```python
from build123d import *

# Parameters (mm, degrees)
SKETCH1_W           = 620
SKETCH1_H           = 680
BOSS_EXTRUDE1_DEPTH = 15
SKETCH2_R           = 4
CUT_EXTRUDE1_DEPTH  = 10
LPATTERN1_COUNT     = 3
LPATTERN1_PITCH     = 295
SKETCH3_R           = 4
CUT_EXTRUDE2_DEPTH  = 10
LPATTERN2_COUNT     = 3
LPATTERN2_PITCH     = 325
SKETCH7_R           = 4
CUT_EXTRUDE7_DEPTH  = 10
SKETCH8_W           = 10
SKETCH8_H           = 20
CUT_EXTRUDE8_DEPTH  = 435


with BuildPart() as part:
    # Sketch1 → Boss-Extrude1 (new body)
    with BuildSketch(Plane(origin=(0, 0, 0), x_dir=(0, 0, -1), z_dir=(1, 0, 0))):
        with Locations((0, 340)):
            Rectangle(SKETCH1_W, SKETCH1_H)
    extrude(amount=BOSS_EXTRUDE1_DEPTH)

    # Sketch2 → Cut-Extrude1 (cut)
    with BuildSketch(Plane.ZY):
        with Locations((295, 7.5)):
            Circle(SKETCH2_R)
    cut_extrude1 = extrude(amount=-CUT_EXTRUDE1_DEPTH, mode=Mode.SUBTRACT)

    # LPattern1: Cut-Extrude1 ×3
    with Locations(*[(0, 0, -i * LPATTERN1_PITCH) for i in range(1, LPATTERN1_COUNT)]):
        add(cut_extrude1, mode=Mode.SUBTRACT)

    # Sketch3 → Cut-Extrude2 (cut)
    with BuildSketch(Plane(origin=(0, 0, -310), x_dir=(-1, 0, 0), z_dir=(0, 0, -1))):
        with Locations((-7.5, 15)):
            Circle(SKETCH3_R)
    cut_extrude2 = extrude(amount=-CUT_EXTRUDE2_DEPTH, mode=Mode.SUBTRACT)

    # LPattern2: Cut-Extrude2 ×3
    with Locations(*[(0, i * LPATTERN2_PITCH, 0) for i in range(1, LPATTERN2_COUNT)]):
        add(cut_extrude2, mode=Mode.SUBTRACT)

    # Sketch7 → Cut-Extrude7 (cut)
    with BuildSketch(Plane.XY.offset(310)):
        with Locations((7.5, 670)):
            Circle(SKETCH7_R)
    extrude(amount=-CUT_EXTRUDE7_DEPTH, mode=Mode.SUBTRACT)

    # Sketch8 → Cut-Extrude8 (cut)
    with BuildSketch(Plane(origin=(0, 680, 0), x_dir=(1, 0, 0), z_dir=(0, 1, 0))):
        with Locations((10, -287.5)):
            Rectangle(SKETCH8_W, SKETCH8_H)
    extrude(amount=-CUT_EXTRUDE8_DEPTH, mode=Mode.SUBTRACT)


solid = part.part
```
Can you work these out from the model? Positions are in its coordinate system, mm. Give positions to 0.01 mm unless a question says otherwise; leave off trailing zeros. Write each loop counter-clockwise with the first axis right and the second up, starting at its lowest first coordinate (ties: lowest second). Pieces come first, ordered by that corner, then holes. Notation, with made-up numbers: (-16, 63) - (1, 63) arc R17 ccw to (1, 80) - close; hole circle Ø10 at (-37, 26.25). An arc over 180 degrees is marked (long way). Write item = value, one per line. Start each with the question number.
1. For pin 1 (7 mm diameter, centred on y = 7.5, z = -295, fed in from -X); pin 2 (2.5 mm diameter, centred on x = 6.5, y = 665, fed in from -Z); pin 3 (8 mm diameter, centred on x = 12, z = 288, fed in from +Y), each with a flat end and sliding along its axis, tell me the tip position at first contact or that it passes through.
2. Please list where these lines run through material, in increasing order: line 1 (Y direction, x = 7.5, z = -305); line 2 (Z direction, x = 10.5, y = 274); line 3 (Y direction, x = 2, z = 0).
3. Imagine slicing it at A-A (y = 269.5). Please give me the cut outline in (x, z), and give its area (3 significant figures).
4. Imagine slicing it at B-B (x = 7.5). Please give me the cut outline in (y, z), and give its area (3 significant figures).
5. Thinking about a two-plate mould opening in Z: for faces 1 (the face through (7, 335, -310)), 2 (the face through (0, 345, 4)), 3 (the face through (5, 466, 288)), which applies, released by +Z, released by -Z, zero draft, split by the parting line, or undercut?
Worked answers:
q1.pin_1 = 10
q1.pin_2 = -300
q1.pin_3 = 245
q2.line_1 = 0 to 11, 19 to 336, 344 to 661, 669 to 680
q2.line_2 = -310 to 277.5, 297.5 to 310
q2.line_3 = 0 to 3.5, 11.5 to 680
q3.outline = (0, -310) - (15, -310) - (15, 277.5) - (5, 277.5) - (5, 297.5) - (15, 297.5) - (15, 310) - (0, 310) - close
q3.area = 9,100 mm2
q4.outline = (0, -310) - (11, -310) - (11, -300) - (19, -300) - (19, -310) - (336, -310) - (336, -300) - (344, -300) - (344, -310) - (661, -310) - (661, -300) - (669, -300) - (669, -310) - (680, -310) - (680, 277.5) - (245, 277.5) - (245, 297.5) - (680, 297.5) - (680, 310) - (674, 310) - (674, 300) - (666, 300) - (666, 310) - (0, 310) - close; hole circle Ø8 at (7.5, -295); hole circle Ø8 at (7.5, 0); hole circle Ø8 at (7.5, 295)
q4.area = 412,000 mm2
q5.face_1 = released by -Z
q5.face_2 = zero draft
q5.face_3 = undercut
